For this review, take the finished solid that the model builds, in its own axes (mm). A direction names the side the tool comes from. Give positions to 0.01 mm unless a question says otherwise; leave off trailing zeros. Loops run counter-clockwise (first coordinate to the right, second up) from the corner with the lowest first, then second, coordinate; pieces in that order, holes last. Notation, with made-up numbers: (-36, -36.75) - (-16, -36.75) arc R34 ccw to (-16, -5.75) - close; hole circle Ø3 at (-10, -38.75). An arc over 180 degrees is marked (long way). Answer in a Markdown table with one row per item.
```python
from build123d import *

# Parameters (mm, degrees)
F1_DEPTH  = 10
F3_DEPTH  = 10
F5_DEPTH  = 10
F7_W      = 10
F7_H      = 10
F8_DEPTH  = 100
F10_DEPTH = 5
F12_DEPTH = 5


with BuildPart() as f1:
    # F0 (on Top) → F1 (new body)
    with BuildSketch(Plane.XY):
        Polygon((-23.817373896, 17.9644496739), (-23.817373896, -22.0355503261), (-13.817373896, -22.0355503261), (-13.817373896, -12.0355503261), (-13.817373896, 7.9644496739), (11.182626104, 7.9644496739), (36.182626104, 7.9644496739), (36.182626104, -12.0355503261), (36.182626104, -22.0355503261), (46.182626104, -22.0355503261), (46.182626104, 17.9644496739), (11.182626104, 17.9644496739), align=None)
    extrude(amount=F1_DEPTH)

    # F2 (on face) → F3 (join)
    with BuildSketch(Plane.YZ.offset(-13.817373896)):
        with BuildLine():
            ThreePointArc((-17.0355503261, 0), (-13.5000164202, 1.4644660941), (-12.0355503261, 5))
            ThreePointArc((-12.0355503261, 5), (-13.5000164202, 8.5355339059), (-17.0355503261, 10))
            ThreePointArc((-17.0355503261, 10), (-20.571084232, 8.5355339059), (-22.0355503261, 5))
            ThreePointArc((-22.0355503261, 5), (-20.571084232, 1.4644660941), (-17.0355503261, 0))
        make_face()
    extrude(amount=F3_DEPTH)

    # F4 (on face) → F5 (join)
    with BuildSketch(Plane(origin=(36.182626104, 0, 0), x_dir=(0, -1, 0), z_dir=(-1, 0, 0))):
        with BuildLine():
            ThreePointArc((17.0355503261, 0), (20.571084232, 1.4644660941), (22.0355503261, 5))
            ThreePointArc((22.0355503261, 5), (20.571084232, 8.5355339059), (17.0355503261, 10))
            ThreePointArc((17.0355503261, 10), (12.0355503261, 5), (17.0355503261, 0))
        make_face()
    extrude(amount=F5_DEPTH)

    # F7 (on face) → F8 (join)
    with BuildSketch(Plane(origin=(0, 8.9822248369, 8.9822248369), x_dir=(1, 0, 0), z_dir=(0, -0.7071067812, -0.7071067812))):
        with Locations((26.182626104, -3.560648561)):
            Rectangle(F7_W, F7_H)
        with Locations((-3.817373896, -3.560648561)):
            Rectangle(F7_W, F7_H)
    extrude(amount=-F8_DEPTH)

    # F9 (on face) → F10 (join)
    with BuildSketch(Plane.YZ.offset(1.182626104)):
        with BuildLine():
            ThreePointArc((82.2106616934, 70.1040763958), (83.2945254537, 71.7261931416), (83.6751277925, 73.6396103068))
            ThreePointArc((83.6751277925, 73.6396103068), (83.2945254551, 75.5530274686), (82.2106616985, 77.1751442127))
            ThreePointArc((82.2106616985, 77.1751442127), (78.6751277925, 78.6396103068), (75.1395938866, 77.1751442127))
            ThreePointArc((75.1395938866, 77.1751442127), (75.1395938841, 70.1040764034), (82.2106616934, 70.1040763958))
        make_face()
    extrude(amount=F10_DEPTH)

    # F11 (on face) → F12 (join)
    with BuildSketch(Plane(origin=(21.182626104, 0, 0), x_dir=(0, -1, 0), z_dir=(-1, 0, 0))):
        with BuildLine():
            ThreePointArc((-82.2106617767, 70.104076479), (-76.7617106818, 69.0202126231), (-73.6751277925, 73.6396103068))
            ThreePointArc((-73.6751277925, 73.6396103068), (-74.0557301241, 75.5530274545), (-75.139593865, 77.1751441911))
            ThreePointArc((-75.139593865, 77.1751441911), (-78.6751277889, 78.6396103068), (-82.210661715, 77.1751441962))
            ThreePointArc((-82.210661715, 77.1751441962), (-83.6751277925, 73.6396103504), (-82.2106617767, 70.104076479))
        make_face()
    extrude(amount=F12_DEPTH)


solid = f1.part
```
1. Clearance check with flat-ended pins moving along their axes: pin 1 (12 mm diameter, centred on x = 39, y = -9.5, fed in from +Z); pin 2 (5 mm diameter, centred on y = 80, z = 74.5, fed in from -X); pin 3 (12 mm diameter, centred on x = 24, z = 63, fed in from -Y). State where each tip first meets the part, or that it passes through.
Values:
| item | result |
|---|---|
| pin 1 | stops at z = 10 |
| pin 2 | stops at x = -8.82 |
| pin 3 | stops at y = 54.96 |
2. We need section A-A, the plane x = -7.5. Give the boundary of the cut face in (y, z).
Values:
| item | result |
|---|---|
| outline | circle Ø10 at (-17.04, 5); (7.96, 0) - (17.96, 0) - (17.96, 5.86) - (85.75, 73.64) - (78.68, 80.71) - (7.96, 10) - close |
3. Wall thickness on line 1 (X direction, y = 70.5, z = 61); line 2 (Z direction, x = -19, y = -11); line 3 (Y direction, x = -8, z = 39.5): over which ranges is each line inside the solid? List them lowest first. Write a range as [from, to].
Values:
| item | result |
|---|---|
| line 1 | x = [-8.82, 1.18], [21.18, 31.18] |
| line 2 | z = [0, 10] |
| line 3 | y = [37.46, 51.61] |
4. Mouldability with a two-part tool opening along X and no side actions: class faces 1 (the face through (26.113, 82.161, 77.225)), 2 (the face through (16.183, 79, 74)) as released by +X, released by -X, zero draft, split by the parting line, or undercut.
Values:
| item | result |
|---|---|
| face 1 | zero draft |
| face 2 | undercut |
5. For faces 3 (the face through (-3.817, -17, 5)), 4 (the face through (36.183, -21, 1)), 5 (the face through (11, 13, 10)), list the 3-axis set-ups (+Z, -Z, +X, -X, +Y, -Y) from which the entire face can be reached by the end or side of a thin tool; tool diameter is ignored.
Values:
| item | result |
|---|---|
| face 3 | +Z, -Z, -Y |
| face 4 | -Z, -Y |
| face 5 | +Z, +Y, -Y |
6. We need section C-C, the plane z = 38. Give the boundary of the cut face in (x, y), and give its area (3 significant figures).
Values:
| item | result |
|---|---|
| outline | (-8.82, 35.96) - (1.18, 35.96) - (1.18, 50.11) - (-8.82, 50.11) - close; (21.18, 35.96) - (31.18, 35.96) - (31.18, 50.11) - (21.18, 50.11) - close |
| area | 283 mm^2 |
7. We need section B-B, the plane y = -1.5. Give the boundary of the cut face in (x, z), and give its area (3 significant figures).
Values:
| item | result |
|---|---|
| outline | (-23.82, 0) - (-13.82, 0) - (-13.82, 10) - (-23.82, 10) - close; (36.18, 0) - (46.18, 0) - (46.18, 10) - (36.18, 10) - close |
| area | 200 mm^2 |
